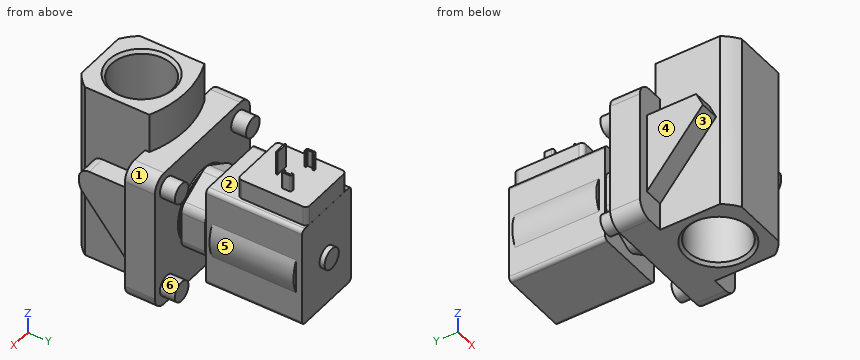
```python
from build123d import *

# Parameters (mm, degrees)
IZIM1_W                      = 50.7
IZIM1_H                      = 48.2
Y_KSEKLIK_EKSTR_ZYON1_DEPTH  = 26.7
IZIM2_R                      = 8.7
Y_KSEKLIK_EKSTR_ZYON2_DEPTH  = 0.5
Y_KSEKLIK_EKSTR_ZYON3_DEPTH  = 11.9
IZIM4_R                      = 16.5
Y_KSEKLIK_EKSTR_ZYON4_DEPTH  = 0.9
IZIM5_R                      = 18
Y_KSEKLIK_EKSTR_ZYON5_DEPTH  = 0.9
Y_KSEKLIK_EKSTR_ZYON6_DEPTH  = 36
Y_KSEKLIK_EKSTR_ZYON7_DEPTH  = 17
Y_KSEKLIK_EKSTR_ZYON8_START  = 17
Y_KSEKLIK_EKSTR_ZYON8_DEPTH  = 17
IZIM9_W                      = 14.75
IZIM9_H                      = 70
KES_EKSTR_ZYON1_DEPTH        = 30.160746911
IZIM10_W                     = 14.75
IZIM10_H                     = 70
KES_EKSTR_ZYON2_DEPTH        = 30.160746911
IZIM11_W                     = 50.7
IZIM11_H                     = 48.2
Y_KSEKLIK_EKSTR_ZYON9_DEPTH  = 9.3
Y_KSEKLIK_EKSTR_ZYON10_START = 20
Y_KSEKLIK_EKSTR_ZYON10_DEPTH = 20
IZIM13_W                     = 9.75
IZIM13_H                     = 10.2
Y_KSEKLIK_EKSTR_ZYON11_DEPTH = 26.5
Y_KSEKLIK_EKSTR_ZYON12_DEPTH = 42.2
Y_KSEKLIK_EKSTR_ZYON13_START = -42.2
Y_KSEKLIK_EKSTR_ZYON13_DEPTH = 42.2
IZIM16_W                     = 29
IZIM16_H                     = 34.79
Y_KSEKLIK_EKSTR_ZYON14_DEPTH = 9.9
Y_KSEKLIK_EKSTR_ZYON15_DEPTH = 8.5
Y_KSEKLIK_EKSTR_ZYON16_DEPTH = 8.5
IZIM19_W                     = 6.3
IZIM19_H                     = 0.8
Y_KSEKLIK_EKSTR_ZYON17_DEPTH = 12
DRAFT1_ANGLE                 = 50
IZIM20_W                     = 5
IZIM20_H                     = 7.5
IZIM21_W                     = 5
IZIM21_H                     = 7.5
IZIM22_W                     = 5
IZIM22_H                     = 7.5
IZIM23_W                     = 5
IZIM23_H                     = 7.5
IZIM24_W                     = 5.2
IZIM24_H                     = 2.6
M27_BO_LUKLU_DELIK1_D        = 30.291
M27_BO_LUKLU_DELIK1_DEPTH    = 33.249
M27_BO_LUKLU_DELIK2_D        = 30.291
M27_BO_LUKLU_DELIK2_DEPTH    = 33.249
FEDER1_START                 = -30
FEDER1_DEPTH                 = 9.75
PAH1_SIZE                    = 1.479
RADYUS1_R                    = 0.8
RADYUS2_R                    = 2
RADYUS3_R                    = 5
RADYUS4_R                    = 5.1
RADYUS5_R                    = 7
RADYUS6_R                    = 8.16
L_EK1_SCALE                  = 0.27


# Read off the part's stored shape, not the designer's step: Feder1
with BuildPart() as part:
    # Çizim1 → Yükseklik-Ekstrüzyon1 (new body)
    with BuildSketch(Plane(origin=(18, 0, 0), x_dir=(0, 0, -1), z_dir=(1, 0, 0))):
        with Locations((-0.35, 68.8)):
            Rectangle(IZIM1_W, IZIM1_H)
    extrude(amount=-Y_KSEKLIK_EKSTR_ZYON1_DEPTH)

    # Çizim2 → Yükseklik-Ekstrüzyon2 (add)
    with BuildSketch(Plane.XZ.offset(-44.7)):
        with Locations(Location((0, 0, 0), (0, 0, 180))):
            Circle(IZIM2_R)
    extrude(amount=Y_KSEKLIK_EKSTR_ZYON2_DEPTH)

    # Çizim3 → Yükseklik-Ekstrüzyon3 (add)
    with BuildSketch(Plane(origin=(0, 44.2, 0), x_dir=(1, 0, 0), z_dir=(0, 1, 0))):
        Polygon((-18, 10.392304845), (-18, -10.392304845), (0, -20.784609691), (18, -10.392304845), (18, 10.392304845), (0, 20.784609691), align=None)
    extrude(amount=-Y_KSEKLIK_EKSTR_ZYON3_DEPTH)

    # Çizim4 → Yükseklik-Ekstrüzyon4 (add)
    with BuildSketch(Plane.XZ.offset(-32.3)):
        with Locations(Location((0, 0, 0), (0, 0, 270))):
            Circle(IZIM4_R)
    extrude(amount=Y_KSEKLIK_EKSTR_ZYON4_DEPTH)

    # Çizim5 → Yükseklik-Ekstrüzyon5 (add)
    with BuildSketch(Plane(origin=(0, 31.4, 0), x_dir=(1, 0, 0), z_dir=(0, 1, 0))):
        with Locations(Location((0, 0, 0), (0, 0, 90))):
            Circle(IZIM5_R)
    extrude(amount=-Y_KSEKLIK_EKSTR_ZYON5_DEPTH)

    # Çizim6 → Yükseklik-Ekstrüzyon6 (add)
    with BuildSketch(Plane.XY.offset(18)):
        with BuildLine():
            Line((-13.564659966, -21), (13.564659966, -21))
            ThreePointArc((13.564659966, -21), (17.201870235, -18.14099392), (20.25, -14.660746911))
            Line((20.25, -14.660746911), (35, -14.660746911))
            Line((35, -14.660746911), (35, 30.5))
            Line((35, 30.5), (0, 30.5))
            Line((0, 30.5), (-35, 30.5))
            Line((-35, 30.5), (-35, -14.660746911))
            Line((-35, -14.660746911), (-20.25, -14.660746911))
            ThreePointArc((-20.25, -14.660746911), (-17.201870235, -18.14099392), (-13.564659966, -21))
        make_face()
    extrude(amount=-Y_KSEKLIK_EKSTR_ZYON6_DEPTH)

    # Çizim7 → Yükseklik-Ekstrüzyon7 (add)
    with BuildSketch(Plane(origin=(0, 0, -18), x_dir=(-1, 0, 0), z_dir=(0, 0, -1))):
        with BuildLine():
            Line((13.564659966, -21), (-13.564659966, -21))
            ThreePointArc((-13.564659966, -21), (-17.201870235, -18.14099392), (-20.25, -14.660746911))
            Line((-20.25, -14.660746911), (-35, -14.660746911))
            Line((-35, -14.660746911), (-35, 30.5))
            Line((-35, 30.5), (35, 30.5))
            Line((35, 30.5), (35, -14.660746911))
            Line((35, -14.660746911), (20.25, -14.660746911))
            ThreePointArc((20.25, -14.660746911), (17.201870235, -18.14099392), (13.564659966, -21))
        make_face()
    extrude(amount=Y_KSEKLIK_EKSTR_ZYON7_DEPTH)

    # Çizim8 → Yükseklik-Ekstrüzyon8 (add)
    with BuildSketch(Plane.XY.offset(18).offset(Y_KSEKLIK_EKSTR_ZYON8_START)):
        with BuildLine():
            Line((13.564659966, -21), (-13.564659966, -21))
            ThreePointArc((-13.564659966, -21), (-17.201870235, -18.14099392), (-20.25, -14.660746911))
            Line((-20.25, -14.660746911), (-35, -14.660746911))
            Line((-35, -14.660746911), (-35, 30.5))
            Line((-35, 30.5), (35, 30.5))
            Line((35, 30.5), (35, -14.660746911))
            Line((35, -14.660746911), (20.25, -14.660746911))
            ThreePointArc((20.25, -14.660746911), (17.201870235, -18.14099392), (13.564659966, -21))
        make_face()
    extrude(amount=-Y_KSEKLIK_EKSTR_ZYON8_DEPTH)

    # Çizim9 → Kes-Ekstrüzyon1 (cut)
    with BuildSketch(Plane.XZ.offset(14.660746911)):
        with Locations((27.625, 0)):
            Rectangle(IZIM9_W, IZIM9_H)
    extrude(amount=-KES_EKSTR_ZYON1_DEPTH, mode=Mode.SUBTRACT)

    # Çizim10 → Kes-Ekstrüzyon2 (cut)
    with BuildSketch(Plane.XZ.offset(14.660746911)):
        with Locations((-27.625, 0)):
            Rectangle(IZIM10_W, IZIM10_H)
    extrude(amount=-KES_EKSTR_ZYON2_DEPTH, mode=Mode.SUBTRACT)

    # Çizim11 → Yükseklik-Ekstrüzyon9 (add)
    with BuildSketch(Plane.ZY.offset(8.7)):
        with Locations((0.35, 68.8)):
            Rectangle(IZIM11_W, IZIM11_H)
    extrude(amount=Y_KSEKLIK_EKSTR_ZYON9_DEPTH)

    # Çizim12 → Yükseklik-Ekstrüzyon10 (add)
    with BuildSketch(Plane.XY.offset(35).offset(Y_KSEKLIK_EKSTR_ZYON10_START)):
        with BuildLine():
            Line((-20.25, -14.660746911), (-20.25, 17.715834237))
            ThreePointArc((-20.25, 17.715834237), (0, 22), (20.25, 17.715834237))
            Line((20.25, 17.715834237), (20.25, -14.660746911))
            ThreePointArc((20.25, -14.660746911), (17.201870235, -18.14099392), (13.564659966, -21))
            Line((13.564659966, -21), (-13.564659966, -21))
            ThreePointArc((-13.564659966, -21), (-17.201870235, -18.14099392), (-20.25, -14.660746911))
        make_face()
    extrude(amount=-Y_KSEKLIK_EKSTR_ZYON10_DEPTH)

    # Çizim13 → Yükseklik-Ekstrüzyon11 (add)
    with BuildSketch(Plane.XZ.offset(-15.5)):
        with Locations((25.125, 15.1)):
            Rectangle(IZIM13_W, IZIM13_H)
    extrude(amount=Y_KSEKLIK_EKSTR_ZYON11_DEPTH)

    # Çizim14 → Yükseklik-Ekstrüzyon12 (add)
    with BuildSketch(Plane(origin=(0, 89.9, 0), x_dir=(1, 0, 0), z_dir=(0, 1, 0))):
        with BuildLine():
            Line((-18, -8.717797887), (-18, 8.717797887))
            ThreePointArc((-18, 8.717797887), (-20, 0), (-18, -8.717797887))
        make_face()
    extrude(amount=-Y_KSEKLIK_EKSTR_ZYON12_DEPTH)

    # Çizim15 → Yükseklik-Ekstrüzyon13 (add)
    with BuildSketch(Plane.XZ.offset(-47.7).offset(Y_KSEKLIK_EKSTR_ZYON13_START)):
        with BuildLine():
            Line((18, 8.717797887), (18, -8.717797887))
            ThreePointArc((18, -8.717797887), (20, 0), (18, 8.717797887))
        make_face()
    extrude(amount=Y_KSEKLIK_EKSTR_ZYON13_DEPTH)

    # Çizim16 → Yükseklik-Ekstrüzyon14 (add)
    with BuildSketch(Plane.XY.offset(25.7)):
        with Locations((0, 75.495)):
            Rectangle(IZIM16_W, IZIM16_H)
    extrude(amount=Y_KSEKLIK_EKSTR_ZYON14_DEPTH)

    # Çizim17 → Yükseklik-Ekstrüzyon15 (add)
    with BuildSketch(Plane.XY.offset(35.6)):
        Polygon((-9.4, 81.4), (-7.6, 81.4), (-7.6, 80.6), (-8.6, 80.6), (-8.6, 77.4), (-7.6, 77.4), (-7.6, 76.6), (-9.4, 76.6), align=None)
    extrude(amount=Y_KSEKLIK_EKSTR_ZYON15_DEPTH)

    # Çizim18 → Yükseklik-Ekstrüzyon16 (add)
    with BuildSketch(Plane.XY.offset(35.6)):
        Polygon((7.6, 77.4), (8.6, 77.4), (8.6, 80.6), (7.6, 80.6), (7.6, 81.4), (9.4, 81.4), (9.4, 76.6), (7.6, 76.6), align=None)
    extrude(amount=Y_KSEKLIK_EKSTR_ZYON16_DEPTH)

    # Çizim19 → Yükseklik-Ekstrüzyon17 (add)
    with BuildSketch(Plane.XY.offset(35.6)):
        with Locations((0, 70)):
            Rectangle(IZIM19_W, IZIM19_H)
    extrude(amount=Y_KSEKLIK_EKSTR_ZYON17_DEPTH)

    # Draft1
    draft1_faces = [part.faces().sort_by_distance(p)[0] for p in [
        (25.125, 2.25, 10),
    ]]
    draft(draft1_faces, Plane(origin=(0, -11, 0), x_dir=(0, 0, -1), z_dir=(0, -1, 0)), DRAFT1_ANGLE)

    # Çizim20 → Döndür1 (revolve)
    with BuildSketch(Plane.XY.offset(26.25), mode=Mode.PRIVATE) as d_nd_r1_sk:
        with Locations((-23.75, 34.25)):
            Rectangle(IZIM20_W, IZIM20_H)
    revolve(d_nd_r1_sk.sketch.rotate(Axis((-26.25, 38, 26.25), (0, -1, 0)), 270), axis=Axis((-26.25, 38, 26.25), (0, -1, 0)))

    # Çizim21 → Döndür2 (revolve)
    with BuildSketch(Plane.XY.offset(-26.25), mode=Mode.PRIVATE) as d_nd_r2_sk:
        with Locations((-23.75, 34.25)):
            Rectangle(IZIM21_W, IZIM21_H)
    revolve(d_nd_r2_sk.sketch.rotate(Axis((-26.25, 38, -26.25), (0, -1, 0)), 270), axis=Axis((-26.25, 38, -26.25), (0, -1, 0)))

    # Çizim22 → Döndür3 (revolve)
    with BuildSketch(Plane.XY.offset(-26.25), mode=Mode.PRIVATE) as d_nd_r3_sk:
        with Locations((28.75, 34.25)):
            Rectangle(IZIM22_W, IZIM22_H)
    revolve(d_nd_r3_sk.sketch.rotate(Axis((26.25, 38, -26.25), (0, -1, 0)), 270), axis=Axis((26.25, 38, -26.25), (0, -1, 0)))

    # Çizim23 → Döndür4 (revolve)
    with BuildSketch(Plane.XY.offset(26.25), mode=Mode.PRIVATE) as d_nd_r4_sk:
        with Locations((28.75, 34.25)):
            Rectangle(IZIM23_W, IZIM23_H)
    revolve(d_nd_r4_sk.sketch.rotate(Axis((26.25, 38, 26.25), (0, -1, 0)), 270), axis=Axis((26.25, 38, 26.25), (0, -1, 0)))

    # Çizim24 → Döndür5 (revolve)
    with BuildSketch(Plane(origin=(0, 0, 0), x_dir=(-1, 0, 0), z_dir=(0, 0, -1)), mode=Mode.PRIVATE) as d_nd_r5_sk:
        with Locations((-2.6, 94.2)):
            Rectangle(IZIM24_W, IZIM24_H)
    revolve(d_nd_r5_sk.sketch.rotate(Axis((0, 92.9, 0), (0, 1, 0)), 90), axis=Axis((0, 92.9, 0), (0, 1, 0)))

    # M27 Boşluklu Delik1
    with Locations(Plane.XY.offset(55)):
        with Locations((0, 0)):
            Hole(M27_BO_LUKLU_DELIK1_D / 2, depth=M27_BO_LUKLU_DELIK1_DEPTH)

    # M27 Boşluklu Delik2
    with Locations(Plane(origin=(0, 0, -35), x_dir=(-1, 0, 0), z_dir=(0, 0, -1))):
        with Locations((0, 0)):
            Hole(M27_BO_LUKLU_DELIK2_D / 2, depth=M27_BO_LUKLU_DELIK2_DEPTH)

    # Feder1 outline → Feder1 (add)
    with BuildSketch(Plane.YZ.offset(FEDER1_START)):
        Polygon((15.5, 19.826070485), (-9.313312955, 19.826070485), (-12.686687045, 12.591846402), (15.5, -20.999739147), align=None)
    extrude(amount=FEDER1_DEPTH)

    # Pah1
    pah1_edges = [part.edges().sort_by_distance(p)[0] for p in [
        (15.1455, 0, 55),
        (-15.1455, 0, -35),
    ]]
    chamfer(pah1_edges, length=PAH1_SIZE)

    # Radyus1
    radyus1_edges = [part.edges().sort_by_distance(p)[0] for p in [
        (-9.4, 81.4, 39.85),
        (-9.4, 76.6, 39.85),
        (9.4, 76.6, 39.85),
        (9.4, 81.4, 39.85),
    ]]
    fillet(radyus1_edges, radius=RADYUS1_R)

    # Radyus2
    radyus2_edges = [part.edges().sort_by_distance(p)[0] for p in [
        (-18, 68.8, -25),
        (-18, 68.8, 25.7),
        (-14.5, 92.89, 30.65),
        (-14.5, 58.1, 30.65),
        (14.5, 58.1, 30.65),
        (14.5, 92.89, 30.65),
        (18, 68.8, 25.7),
        (18, 68.8, -25),
    ]]
    fillet(radyus2_edges, radius=RADYUS2_R)

    # Radyus3
    radyus3_edges = [part.edges().sort_by_distance(p)[0] for p in [
        (-18, 38.25, -10.392304845),
        (0, 38.25, -20.784609691),
        (18, 38.25, -10.392304845),
        (18, 38.25, 10.392304845),
        (0, 38.25, 20.784609691),
        (-18, 38.25, 10.392304845),
    ]]
    fillet(radyus3_edges, radius=RADYUS3_R)

    # Radyus4
    radyus4_edges = [part.edges().sort_by_distance(p)[0] for p in [
        (25.125, -11, 20.2),
    ]]
    fillet(radyus4_edges, radius=RADYUS4_R)

    # Radyus5
    radyus5_edges = [part.edges().sort_by_distance(p)[0] for p in [
        (35, 23, 35),
        (-35, 23, -35),
        (35, 23, -35),
        (-35, 23, 35),
    ]]
    fillet(radyus5_edges, radius=RADYUS5_R)

    # Radyus6
    radyus6_edges = [part.edges().sort_by_distance(p)[0] for p in [
        (25.125, -11, 10),
    ]]
    fillet(radyus6_edges, radius=RADYUS6_R)


with BuildPart() as part_1:
    # Ölçek1: scaled about (0.014445195, 31.538640435, 4.897050437)
    add(part.part.scale(L_EK1_SCALE).moved(Location((0.010544992, 23.023207518, 3.574846819))))


solid = part_1.part
```
Geometry check sheet. Reference: the model listing, model coordinates, mm. Face numbers are marked on the shaded views. A direction names the side the tool comes from. Coordinates: 2 decimals unless noted, no trailing zeros. Loops run counter-clockwise (first coordinate to the right, second up) from the corner with the lowest first, then second, coordinate; pieces in that order, holes last.
Item 1: Go/stop test with flat-tipped pins: pin 1 Ø1 at (y, z) = (44.5, 8) entering from -X; pin 2 Ø0.8 at (x, y) = (7.5, 24) entering from +Z; pin 3 Ø10 at (x, z) = (1.5, -3) entering from +Y. Record where each tip stops, or that it passes through.
Item 2: Access from +Z, -Z, +X, -X, +Y, -Y to the whole of each face (thin tool, end or side, straight path). Record for the marked faces 4, 5 and 6.
Item 3: Release check for a two-part mould opening along Y. For the marked faces 1, 2 and 3 record: released by +Y, released by -Y, zero draft, split by the parting line, or undercut.
Item 4: Sectioned sample at B-B, the plane y = 37. Record the boundary of the cut face in (x, z), then the cut area to 3 significant figures.
Item 5: Sectioned sample at A-A, the plane z = 0.75. Count the separate pieces of the cut face and the enclosed holes in it, then the cut area to 3 significant figures.
Item 6: Thickness scan on line 1 (Y direction, x = -2, z = 8.5); line 2 (Z direction, x = 0.5, y = 47.5); line 3 (X direction, y = 24.5, z = 5.5). Record the ranges inside material, lowest first.
Check result:
1. pin 1: stops at x = -4.85
1. pin 2: stops at z = 9.03
1. pin 3: stops at y = 48.11
2. face 4: +Z, -Z, -X, -Y
2. face 5: +X, +Y
2. face 6: +Y
3. face 1: zero draft
3. face 2: undercut
3. face 3: released by -Y
4. outline: (-4.85, -2.64) arc R0.54 ccw to (-4.31, -3.18) - (4.33, -3.18) arc R0.54 ccw to (4.87, -2.64) - (4.87, 1.22) arc R5.4 ccw to (4.87, 5.93) - (4.87, 9.97) arc R0.54 ccw to (4.33, 10.51) - (-4.31, 10.51) arc R0.54 ccw to (-4.85, 9.97) - (-4.85, 5.93) arc R5.4 ccw to (-4.85, 1.22) - close
4. area: 136 mm2
5. separate pieces: 2
5. enclosed holes: 1
5. area: 302 mm2
6. line 1: y = 17.35 to 31.26, 35.09 to 48.11
6. line 2: z = -3.18 to 13.19
6. line 3: x = -8.09 to 8.11
